```python
from build123d import *

# Parameters (mm, degrees)
PAD_DEPTH       = 2
SKETCH001_R     = 0.5
POCKET_DEPTH    = 5
SKETCH002_W     = 59
SKETCH002_H     = 28
PAD001_DEPTH    = 2
SKETCH003_W     = 28
SKETCH003_H     = 2
PAD002_DEPTH    = 4
CHAMFER_SIZE    = 1
CHAMFER001_SIZE = 1


with BuildPart() as part:
    # Sketch → Pad (new body)
    with BuildSketch(Plane.XY):
        with BuildLine():
            Line((0, 0), (61, 0))
            Line((61, 0), (61, 11.82))
            ThreePointArc((61, 11.82), (64, 14.82), (61, 17.82))
            Line((61, 29.64), (61, 17.82))
            Line((61, 29.64), (0, 29.64))
            Line((0, 29.64), (0, 0))
        make_face()
    extrude(amount=PAD_DEPTH)

    # Sketch001 (on Face7 of Pad) → Pocket (cut)
    with BuildSketch(Plane(origin=(0, 0, 0), x_dir=(1, 0, 0), z_dir=(0, 0, -1))):
        with Locations((61, -14.82)):
            Circle(SKETCH001_R)
    extrude(amount=-POCKET_DEPTH, mode=Mode.SUBTRACT)

    # Sketch002 (on Face4 of Pocket) → Pad001 (join)
    with BuildSketch(Plane(origin=(0, 0, 0), x_dir=(1, 0, 0), z_dir=(0, 0, -1))):
        with Locations((30.5, -15)):
            Rectangle(SKETCH002_W, SKETCH002_H)
    extrude(amount=PAD001_DEPTH)

    # Sketch003 (on Face13 of Pad001) → Pad002 (join)
    with BuildSketch(Plane(origin=(1, 0, 0), x_dir=(0, -1, 0), z_dir=(-1, 0, 0))):
        with Locations((-15, -1)):
            Rectangle(SKETCH003_W, SKETCH003_H)
    extrude(amount=PAD002_DEPTH)

    # Chamfer
    chamfer_edges = [part.edges().sort_by_distance(p)[0] for p in [
        (-3, 1, -1),
        (-3, 29, -1),
        (-3, 15, -2),
    ]]
    chamfer(chamfer_edges, length=CHAMFER_SIZE)

    # Chamfer001
    chamfer001_edges = [part.edges().sort_by_distance(p)[0] for p in [
        (60.5, 14.82, 2),
    ]]
    chamfer(chamfer001_edges, length=CHAMFER001_SIZE)


solid = part.part
```
Read the model definition and answer for the solid it produces. Units are mm, in the model's axes. A direction names the side the tool comes from. Coordinates: 2 decimals unless noted, no trailing zeros. Loops run counter-clockwise (first coordinate to the right, second up) from the corner with the lowest first, then second, coordinate; pieces in that order, holes last.
(1) The part is cut by section A-A (y = 11). Determine the outline of the cut face in (x, z).
Solution:
outline: (-3, -1) - (-2, -2) - (60, -2) - (60, 0) - (61, 0) - (61, 2) - (0, 2) - (0, 0) - (-3, 0) - close
(2) Consider line 1 along X through (y, z) = (14.82, 0.5); line 2 along X through (y, z) = (8.25, 0.55); line 3 along X through (y, z) = (13.25, -0.85). Determine where each line is inside the solid, lowest interval first.
Solution:
line 1: x = 0 to 60.5, 61.5 to 64
line 2: x = 0 to 61
line 3: x = -3 to 60
(3) Flat-ended cylindrical pins translate along their axes: pin 1 Ø2 at (y, z) = (26.5, 0.5) entering from +X; pin 2 Ø1.6 at (y, z) = (12, -1) entering from +X; pin 3 Ø0.6 at (x, z) = (40.5, -1) entering from +Y. Find the tip coordinate at first contact, or state that the pin passes through.
Solution:
pin 1: stops at x = 61
pin 2: stops at x = 60
pin 3: stops at y = 29
(4) The part is cut by section B-B (x = 53.5). Determine the outline of the cut face in (y, z), and give its area (3 significant figures).
Solution:
outline: (0, 0) - (1, 0) - (1, -2) - (29, -2) - (29, 0) - (29.64, 0) - (29.64, 2) - (0, 2) - close
area: 115 mm2
(5) A tool of negligible diameter and unlimited length cuts with its end or side. For faces 1 (the face through (60, 15, -1)), 2 (the face through (29, 1, -1)), 3 (the face through (0, 15, 1)), 4 (the face through (61, 24, 1)), from which of +Z, -Z, +X, -X, +Y, -Y can it reach the whole face along a straight path? Write none if from no direction.
Solution:
face 1: -Z, +X, +Y, -Y
face 2: -Z, +X, -X, -Y
face 3: +Z, -X, +Y, -Y
face 4: +Z, -Z, +X, +Y
